```python
from build123d import *

# Parameters (mm, degrees)
SKETCH1_R                = 6.35
SKETCH1_R_2              = 3.175
BOSS_EXTRUDE1_DEPTH      = 22.5
SKETCH1_3_R              = 3.175
SKETCH1_3_R_2            = 3
BOSS_EXTRUDE2_DEPTH      = 7
BOSS_EXTRUDE3_DEPTH      = 6.35
BOSS_EXTRUDE3_DEPTH_BACK = 6.35
SKETCH3_W                = 6.35
SKETCH3_H                = 2.286
BOSS_EXTRUDE4_DEPTH      = 3.175
BOSS_EXTRUDE4_DEPTH_BACK = 3.175
SKETCH3_4_W              = 6.35
SKETCH3_4_H              = 2.286
SKETCH1_4_R              = 3
CUT_EXTRUDE2_DEPTH       = 33.697891369
FILLET1_R                = 6.35


with BuildPart() as part:
    # Sketch1 → Boss-Extrude1 (new body)
    with BuildSketch(Plane.YZ):
        with Locations(Location((0, 0, 0), (0, 0, 90))):
            Circle(SKETCH1_R)
        with Locations(Location((0, 0, 0), (0, 0, 90))):
            Circle(SKETCH1_R_2, mode=Mode.SUBTRACT)
    extrude(amount=BOSS_EXTRUDE1_DEPTH)

    # Sketch1<3> → Boss-Extrude2 (add)
    with BuildSketch(Plane.YZ):
        with Locations(Location((0, 0, 0), (0, 0, 90))):
            Circle(SKETCH1_3_R)
        with Locations(Location((0, 0, 0), (0, 0, 270))):
            Circle(SKETCH1_3_R_2, mode=Mode.SUBTRACT)
    extrude(amount=BOSS_EXTRUDE2_DEPTH)

    # Sketch3 → Boss-Extrude3 (add, two sides: drawn at the far end of the back side and taken through both)
    with BuildSketch(Plane(origin=(0, 0, 0), x_dir=(0, 1, 0), z_dir=(0, 0, 1)).offset(-BOSS_EXTRUDE3_DEPTH_BACK)):
        Polygon((0, -2.286), (0, 0), (-22.86, 0), (-22.86, -2.286), (-16.51, -2.286), align=None)
        with Locations((-19.685, -5.715)):
            Rectangle(SKETCH3_W, SKETCH3_H)
    extrude(amount=BOSS_EXTRUDE3_DEPTH + BOSS_EXTRUDE3_DEPTH_BACK)


with BuildPart() as boss_extrude3_piece_1:
    # of the separate pieces the step leaves, piece 1, a body of its own (boss_extrude3_pieces)
    add(part.part.solids().sort_by_distance((0, 0, -6.35))[0])



with BuildPart() as boss_extrude3_piece_2:
    # of the separate pieces the step leaves, piece 2, a body of its own (boss_extrude3_pieces)
    add(part.part.solids().sort_by_distance((4.572, -16.51, 6.35))[0])


with BuildPart() as boss_extrude3_piece_1_1:
    add(boss_extrude3_piece_1.part)

    add(boss_extrude3_piece_2.part)  # Boss-Extrude4 merges Boss-Extrude3 piece 2
    # Sketch3<4> → Boss-Extrude4 (add, two sides: drawn at the far end of the back side and taken through both)
    with BuildSketch(Plane(origin=(0, 0, 0), x_dir=(0, 1, 0), z_dir=(0, 0, 1)).offset(-BOSS_EXTRUDE4_DEPTH_BACK)):
        with Locations((-19.685, -3.429)):
            Rectangle(SKETCH3_4_W, SKETCH3_4_H)
    extrude(amount=BOSS_EXTRUDE4_DEPTH + BOSS_EXTRUDE4_DEPTH_BACK)

    # Sketch1<4> → Cut-Extrude2 (cut, through all)
    with BuildSketch(Plane.YZ):
        with Locations(Location((0, 0, 0), (0, 0, 270))):
            Circle(SKETCH1_4_R)
    extrude(amount=CUT_EXTRUDE2_DEPTH, mode=Mode.SUBTRACT)

    # Fillet1
    # the kernel refuses this fillet: 6.35 mm, written as the material it takes off along each edge
    with BuildSketch(Plane(origin=(-15.875, -22.86, -6.35), x_dir=(0, 1, 0), z_dir=(1, 0, 0))) as fillet1_piece_1:
        with BuildLine():
            CenterArc((FILLET1_R, FILLET1_R), FILLET1_R, 180, 90)
            Line((0, FILLET1_R), (0, 0))
            Line((0, 0), (FILLET1_R, 0))
        make_face()
    extrude(amount=34.036, mode=Mode.SUBTRACT)
    with BuildSketch(Plane(origin=(-15.875, -22.86, 6.35), x_dir=(0, 1, 0), z_dir=(1, 0, 0))) as fillet1_piece_2:
        with BuildLine():
            CenterArc((FILLET1_R, -FILLET1_R), FILLET1_R, 90, 90)
            Line((0, -FILLET1_R), (0, 0))
            Line((0, 0), (FILLET1_R, 0))
        make_face()
    extrude(amount=34.036, mode=Mode.SUBTRACT)


solid = boss_extrude3_piece_1_1.part
```
Geometry: final body of the model. Coordinates: model frame, mm. A direction names the side the tool comes from. Coordinates: 2 decimals unless noted, no trailing zeros. Order: outer loops, then holes, each group sorted by start corner. A loop starts at its lowest first (then second) coordinate and runs counter-clockwise, first axis right, second up. Notation, with made-up numbers: (57.5, -13) - (95.5, -13) arc R15 cw to (95.5, 10) - close; hole circle Ø5 at (-1.75, 59). An arc over 180 degrees is marked (long way). Return JSON: item names as keys, results as strings. Group by question number.
1. Pull-direction query (Z, two-part tool) for faces 1 (the face through (11.092, 5.634, 2.93)), 2 (the face through (14.64, 1.93, -2.52)), 3 (the face through (3.45, 0.9, -2.86)), 4 (the face through (22.5, -3, -2)); classes: pulls with the +Z half, pulls with the -Z half, needs draft (parallel to the pull), parting line crosses it, or undercut.
2. Cut plane B-B (z = 0). Output: boundary loops of the cut face in (x, y) (3 decimals).
3. Cut plane C-C (y = 2). Output: boundary loops of the cut face in (x, z), plus the area to 3 significant figures.
4. Cut plane D-D (z = 4.5). Output: boundary loops of the cut face in (x, y), plus the area to 3 significant figures.
5. Cut plane A-A (x = 5.75). Output: boundary loops of the cut face in (y, z), plus the area to 3 significant figures.
6. Set-up query: faces 5 (the face through (3, -19, -3.175)), 6 (the face through (3, -19, 3.175)), 7 (the face through (5, -16.51, 0)). Return all of +Z, -Z, +X, -X, +Y, -Y with unobstructed straight access to the full face (end or side cutting, diameter ignored); none if empty.
7. Pin query (flat end, axial travel): pin 1 (4 mm diameter, centred on x = 12, z = 1, fed in from -Y); pin 2 (3 mm diameter, centred on y = -7.5, z = 4, fed in from +X); pin 3 (2.5 mm diameter, centred on x = 3.5, y = -20.5, fed in from -Z). Return the tip coordinate at first contact, or that it passes through.
8. Material intervals for line 1 along Y through (x, z) = (4, 0); line 2 along Y through (x, z) = (3.25, -1.5); line 3 along Y through (x, z) = (14.5, 0) (3 decimals), sorted ascending. Write a range as [from, to].
Resolved:
{
 "1": {"face 1": "parting line crosses it", "face 2": "undercut", "face 3": "undercut", "face 4": "needs draft"},
 "2": {"outline": "(0, -22.86) - (6.858, -22.86) - (6.858, -16.51) - (2.286, -16.51) - (2.286, -6.35) - (22.5, -6.35) - (22.5, -3.175) - (7, -3.175) - (7, -3) - (0, -3) - close; (0, 3) - (7, 3) - (7, 3.175) - (22.5, 3.175) - (22.5, 6.35) - (0, 6.35) - close"},
 "3": {"outline": "(0, -6.03) - (22.5, -6.03) - (22.5, -2.47) - (7, -2.47) - (7, -2.24) - (0, -2.24) - close; (0, 2.24) - (7, 2.24) - (7, 2.47) - (22.5, 2.47) - (22.5, 6.03) - (0, 6.03) - close", "area": "163 mm²"},
 "4": {"outline": "(0, -20.99) - (2.29, -20.99) - (2.29, -4.48) - (22.5, -4.48) - (22.5, 4.48) - (0, 4.48) - close; (4.57, -20.99) - (6.86, -20.99) - (6.86, -16.51) - (4.57, -16.51) - close", "area": "250 mm²"},
 "5": {"outline": "(-16.51, -6.35) - (-16.51, 6.35) arc R6.35 ccw to start; circle Ø12.7 at (0, 0); hole circle Ø6 at (0, 0)", "area": "162 mm²"},
 "6": {"face 5": "-Z, -Y", "face 6": "+Z, -Y", "face 7": "+Z, -Z, +X"},
 "7": {"pin 1": "stops at y = -6.35", "pin 2": "stops at x = 2.29", "pin 3": "stops at z = -5.4"},
 "8": {"line 1": "y = [-22.86, -16.51], [-6.35, -3], [3, 6.35]", "line 2": "y = [-22.68, -16.51], [-6.17, -2.6], [2.6, 6.17]", "line 3": "y = [-6.35, -3.175], [3.175, 6.35]"}
}
